from build123d import *

# Parameters (mm, degrees)
BOSS_EXTRUDE2_DEPTH = 2.5
SKETCH3_R           = 17.40366437
BOSS_EXTRUDE3_DEPTH = 14
CHAMFER1_SIZE       = 2
CHAMFER1_SIZE2      = 3.200669058
DOME1_FACE_RADIUS   = 14.202995312
DOME1_HEIGHT        = 5.08
SKETCH4_R           = 3.794155
SKETCH4_R_2         = 3.79415255
CUT_EXTRUDE1_DEPTH  = 22.225
FILLET1_R           = 0.5


with BuildPart() as part:
    # Sketch2 → Boss-Extrude2 (new body)
    with BuildSketch(Plane(origin=(0, 0, 0), x_dir=(1, 0, 0), z_dir=(0, 1, 0))):
        with BuildLine():
            Line((-35.297990867, 36.146423133), (-67.605962497, 27.389534463))
            ThreePointArc((-67.605962497, 27.389534463), (-74.11985651, 18.96683835), (-67.783839922, 10.40953043))
            Line((-67.783839922, 10.40953043), (-35.297990867, 4.567846601))
            ThreePointArc((-35.297990867, 4.567846601), (-24.860460433, 1.727880743), (-14.422929998, 4.567846601))
            Line((-14.422929998, 4.567846601), (16.577836549, 10.352015281))
            Line((16.577836549, 10.352015281), (18.329761229, 10.678891968))
            ThreePointArc((18.329761229, 10.678891968), (24.665777818, 19.236199887), (18.151883804, 27.658896001))
            Line((18.151883804, 27.658896001), (-14.156087825, 36.415784671))
            ThreePointArc((-14.156087825, 36.415784671), (-24.766013326, 39.340130463), (-35.297990867, 36.146423133))
        make_face()
    extrude(amount=BOSS_EXTRUDE2_DEPTH)

    # Sketch3 → Boss-Extrude3 (add)
    with BuildSketch(Plane(origin=(0, 2.5, 0), x_dir=(1, 0, 0), z_dir=(0, 1, 0))):
        with Locations((-24.847892724, 20.495392169)):
            Circle(SKETCH3_R)
    extrude(amount=BOSS_EXTRUDE3_DEPTH)

    # Chamfer1
    chamfer1_edges = [part.edges().sort_by_distance(p)[0] for p in [
        (-42.251557093, 16.5, -20.495392169),
    ]]
    chamfer1_side = [part.faces().sort_by_distance(p)[0] for p in [
        (-42.251557093, 9.5, -20.495392169),
    ]]
    chamfer(chamfer1_edges, length=CHAMFER1_SIZE, length2=CHAMFER1_SIZE2, reference=chamfer1_side[0])

    # Dome1: a dome of height H over a round flat face of radius A is a cap of a sphere of radius (A * A + H * H) / (2 * H)
    dome1_r = (DOME1_FACE_RADIUS * DOME1_FACE_RADIUS + DOME1_HEIGHT * DOME1_HEIGHT) / (2 * DOME1_HEIGHT)
    dome1_base = Plane((-24.847892724, 16.5, -20.495392169), z_dir=(0, 1, 0))
    with Locations(dome1_base.offset(DOME1_HEIGHT - dome1_r)):
        dome1_ball = Sphere(dome1_r, mode=Mode.PRIVATE)
    add(split(dome1_ball, bisect_by=dome1_base, keep=Keep.TOP, mode=Mode.PRIVATE))

    # Sketch4 → Cut-Extrude1 (cut)
    with BuildSketch(Plane(origin=(0, 2.5, 0), x_dir=(1, 0, 0), z_dir=(0, 1, 0))):
        with Locations((18.303486059, 18.493262314)):
            Circle(SKETCH4_R)
        with Locations((-68.509987209, 18.493262314)):
            Circle(SKETCH4_R_2)
    extrude(amount=-CUT_EXTRUDE1_DEPTH, mode=Mode.SUBTRACT)

    # Fillet1
    fillet1_edges = [part.edges().sort_by_distance(p)[0] for p in [
        (-42.251557093, 2.5, -20.495392169),
    ]]
    fillet(fillet1_edges, radius=FILLET1_R)


solid = part.part
For this review, take the finished solid that the model builds, in its own axes (mm). A direction names the side the tool comes from. Round coordinates to 2 decimals unless told otherwise and drop trailing zeros. Order: outer loops, then holes, each group sorted by start corner. A loop starts at its lowest first (then second) coordinate and runs counter-clockwise, first axis right, second up. Notation, with made-up numbers: M 29.5,29 L 87.5,29 A18 ccw 87.5,50 Z; hole C -24.75,26 d7. An arc over 180 degrees is marked long. Use a Markdown table: item, result. Add a question column.
Item 1: Mouldability with a two-part tool opening along Z and no side actions: class faces 1 (the cylindrical face through (17.48, 1.27, -14.79)), 2 (the cylindrical face through (-74.117, 1.232, -19.127)), 3 (the flat face through (-28.6, 2.5, -2.5)) as released by +Z, released by -Z, zero draft, split by the parting line, or undercut.
Item 2: Add section A-A, the plane x = -66. Give the boundary of the cut face in (y, z), then the cut area to 3 significant figures.
Item 3: To check wall thickness, follow line 1 along Y through (x, z) = (-4.5, -9); line 2 along X through (y, z) = (2.25, -21); line 3 along X through (y, z) = (14.5, -20). State the ranges of each line that lie inside material, in increasing order.
Item 4: Insertion check: pin 1 (10 mm diameter, centred on y = 14, z = -7, fed in from -X); pin 2 (3 mm diameter, centred on x = -8.5, z = -10, fed in from +Y); pin 3 (2 mm diameter, centred on y = 13.5, z = -20, fed in from -X); pin 4 (7 mm diameter, centred on x = -68.51, z = -18.49, fed in from -Y). Each pin has a flat end and moves straight along its axis. Give the tip position at first contact, or say it passes through.
Item 5: Add section B-B, the plane x = 9.5. Give the boundary of the cut face in (y, z).
Item 6: Tool access review of faces 4 (the flat face through (-51.77, 1.23, -7.53)), 5 (the cylindrical face through (-42.235, 8.67, -21.261)): name each direction out of +Z, -Z, +X, -X, +Y, -Y from which nothing blocks a thin tool from reaching the whole face with its end or side.
Item 7: Add section D-D, the plane x = -46.5. Give the boundary of the cut face in (y, z), then the cut area to 3 significant figures.
Item 8: Add section C-C, the plane y = 13.5. Give the boundary of the cut face in (x, z).
Geometry results:
| question | item | result |
|---|---|---|
| 1 | face 1 | undercut |
| 1 | face 2 | split by the parting line |
| 1 | face 3 | zero draft |
| 2 | outline | M 0,-27.82 L 2.5,-27.82 L 2.5,-21.34 L 0,-21.34 Z; M 0,-15.65 L 2.5,-15.65 L 2.5,-10.09 L 0,-10.09 Z |
| 2 | area | 30.1 mm² |
| 3 | line 1 | y = 0 to 2.5 |
| 3 | line 2 | x = -73.86 to -71.36, -65.66 to 15.46, 21.15 to 24.47 |
| 3 | line 3 | x = -42.24 to -7.45 |
| 4 | pin 1 | stops at x = -40.04 |
| 4 | pin 2 | stops at y = 2.5 |
| 4 | pin 3 | stops at x = -42.25 |
| 4 | pin 4 | passes through |
| 5 | outline | M 0,-30 L 2.5,-30 L 2.5,-9.03 L 0,-9.03 Z |
| 6 | face 4 | +Z, -X, +Y, -Y |
| 6 | face 5 | +Y |
| 7 | outline | M 0,-33.11 L 2.5,-33.11 L 2.5,-6.58 L 0,-6.58 Z |
| 7 | area | 66.3 mm² |
| 8 | outline | C -24.85,-20.5 d34.81 |
